from build123d import *

# Parameters (mm, degrees)
SKETCH1_W           = 60.5
SKETCH1_H           = 75
BOSS_EXTRUDE1_DEPTH = 85.25
SKETCH2_W           = 55
SKETCH2_H           = 165
CUT_EXTRUDE1_DEPTH  = 73.375
SKETCH3_W           = 20
SKETCH3_H           = 10
CUT_EXTRUDE2_DEPTH  = 2.75
SKETCH7_W           = 125
SKETCH7_H           = 10
CUT_EXTRUDE4_DEPTH  = 112.058824503


with BuildPart() as part:
    # Sketch1 → Boss-Extrude1 (new, symmetric)
    with BuildSketch(Plane.XY):
        Rectangle(SKETCH1_W, SKETCH1_H)
    extrude(amount=BOSS_EXTRUDE1_DEPTH, both=True)

    # Sketch2 → Cut-Extrude1 (cut)
    with BuildSketch(Plane(origin=(0, 37.5, 0), x_dir=(1, 0, 0), z_dir=(0, 1, 0))):
        Rectangle(SKETCH2_W, SKETCH2_H)
    extrude(amount=-CUT_EXTRUDE1_DEPTH, mode=Mode.SUBTRACT)

    # Sketch3 → Cut-Extrude2 (cut)
    with BuildSketch(Plane.XY.offset(85.25)):
        with Locations((0, -22.5)):
            Rectangle(SKETCH3_W, SKETCH3_H)
    extrude(amount=-CUT_EXTRUDE2_DEPTH, mode=Mode.SUBTRACT)

    # Sketch7 → Cut-Extrude4 (cut, through all)
    with BuildSketch(Plane.ZY.offset(30.25)):
        with Locations((0, -22.5)):
            Rectangle(SKETCH7_W, SKETCH7_H)
        with Locations((0, 22.5)):
            Rectangle(SKETCH7_W, SKETCH7_H)
    extrude(amount=-CUT_EXTRUDE4_DEPTH, mode=Mode.SUBTRACT)


solid = part.part
Design review of the part built by this model. Coordinates are the model's own, in mm. A direction names the side the tool comes from. Coordinates: 2 decimals unless noted, no trailing zeros. Loops run counter-clockwise (first coordinate to the right, second up) from the corner with the lowest first, then second, coordinate; pieces in that order, holes last. Notation, with made-up numbers: M -7,41.25 L 25,41.25 A22 ccw 25,57.25 Z; hole C -6.75,76 d9. An arc over 180 degrees is marked long. Use one line per item in the form item = value.
(1) Consider section A-A (x = 2). Write out the cut boundary in (y, z) (3 decimals), and give its area (3 significant figures).
Return value:
outline = M -37.5,-85.25 L 37.5,-85.25 L 37.5,-82.5 L -35.875,-82.5 L -35.875,82.5 L -27.5,82.5 L -27.5,85.25 L -37.5,85.25 Z; M -17.5,82.5 L 37.5,82.5 L 37.5,85.25 L -17.5,85.25 Z
area = 653 mm2
(2) Consider section C-C (z = 20). Write out the cut boundary in (x, y) (3 decimals), and give its area (3 significant figures).
Return value:
outline = M -30.25,-37.5 L 30.25,-37.5 L 30.25,-27.5 L 27.5,-27.5 L 27.5,-35.875 L -27.5,-35.875 L -27.5,-27.5 L -30.25,-27.5 Z; M -30.25,-17.5 L -27.5,-17.5 L -27.5,17.5 L -30.25,17.5 Z; M -30.25,27.5 L -27.5,27.5 L -27.5,37.5 L -30.25,37.5 Z; M 27.5,-17.5 L 30.25,-17.5 L 30.25,17.5 L 27.5,17.5 Z; M 27.5,27.5 L 30.25,27.5 L 30.25,37.5 L 27.5,37.5 Z
area = 392 mm2
(3) Consider section B-B (y = 21). Write out the cut boundary in (x, z), and give its area (3 significant figures).
Return value:
outline = M -30.25,-85.25 L 30.25,-85.25 L 30.25,-62.5 L 27.5,-62.5 L 27.5,-82.5 L -27.5,-82.5 L -27.5,-62.5 L -30.25,-62.5 Z; M -30.25,62.5 L -27.5,62.5 L -27.5,82.5 L 27.5,82.5 L 27.5,62.5 L 30.25,62.5 L 30.25,85.25 L -30.25,85.25 Z
area = 553 mm2
(4) For line 1 along Z through (x, y) = (-6.5, -32); line 2 along X through (y, z) = (-27.5, 64.5); line 3 along Y through (x, z) = (3, -32) (3 decimals), list the stretches that pass through material, from the lowest coordinate up. Write a range as from..to.
Return value:
line_1 = -85.25..-82.5, 82.5..85.25
line_2 = -30.25..-27.5, 27.5..30.25
line_3 = -37.5..-35.875
(5) Draft analysis for pull direction Z (two halves, no side actions). For faces 1 (the face through (0, 1, 82.5)), 2 (the face through (0, 1, 85.25)), 3 (the face through (0, -35.875, -1)), 4 (the face through (0, 1, -85.25)), state which applies: pulls with the +Z half, pulls with the -Z half, needs draft (parallel to the pull), parting line crosses it, or undercut.
Return value:
face_1 = undercut
face_2 = pulls with the +Z half
face_3 = undercut
face_4 = pulls with the -Z half
(6) Consider section D-D (y = -2). Write out the cut boundary in (x, z), and give its area (3 significant figures).
Return value:
outline = M -30.25,-85.25 L 30.25,-85.25 L 30.25,85.25 L -30.25,85.25 Z; hole M -27.5,-82.5 L 27.5,-82.5 L 27.5,82.5 L -27.5,82.5 Z
area = 1,240 mm2
(7) Clearance check with flat-ended pins moving along their axes: P1, Ø1, axis at y = -19.5, z = -61, coming from the -X side; P2, Ø6, axis at x = 12, z = -35, coming from the +Y side (3 decimals). State where each tip first meets the part, or that it passes through.
Return value:
P1 = through
P2 = -35.875
(8) For faces 5 (the face through (0, 1, -82.5)), 6 (the face through (0, -37.5, 1)), list the 3-axis set-ups (+Z, -Z, +X, -X, +Y, -Y) from which the entire face can be reached by the end or side of a thin tool; tool diameter is ignored.
Return value:
face_5 = +Y
face_6 = +Z, -Z, +X, -X, -Y
